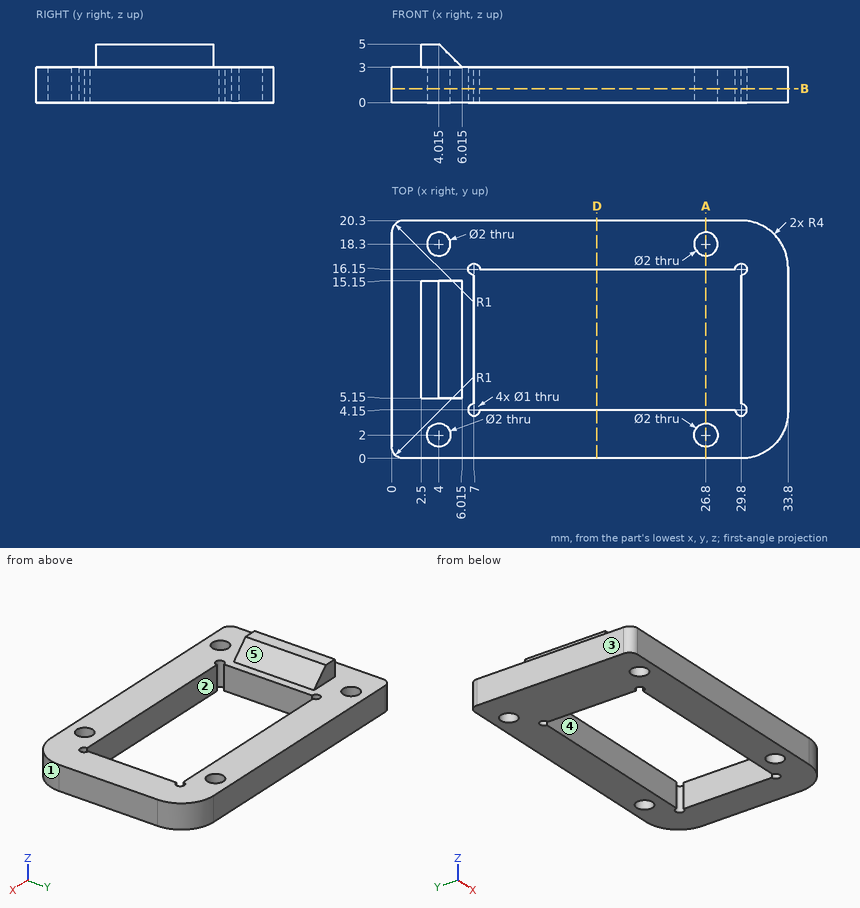
Here's the drawing with two shaded views (mm, measured from the low corner). I have some questions. A direction names the side the tool comes from. Coordinates: 2 decimals unless noted, no trailing zeros. Order: outer loops, then holes, each group sorted by start corner. A loop starts at its lowest first (then second) coordinate and runs counter-clockwise, first axis right, second up.
Item 1: Which directions (+Z, -Z, +X, -X, +Y, -Y) give clear straight access to the entire face, cutting with the end or side of a thin tool? Please do the marked faces 4 and 5.
Response values:
face 4: +Z, -Z
face 5: +Z, +X, +Y, -Y
Item 2: If we section it at A-A, the plane x = 26.8: List the corners of the cut face in (y, z) for me.
Response values:
outline: (0, 0) - (1, 0) - (1, 3) - (0, 3) - close; (3, 0) - (4.15, 0) - (4.15, 3) - (3, 3) - close; (16.15, 0) - (17.3, 0) - (17.3, 3) - (16.15, 3) - close; (19.3, 0) - (20.3, 0) - (20.3, 3) - (19.3, 3) - close
Item 3: I'm going to push flat-ended pins straight in: pin 1 Ø0.6 at (x, z) = (5, 4.5) entering from -Y; pin 2 Ø1 at (x, y) = (23.5, 16.5) entering from +Z; pin 3 Ø0.6 at (x, z) = (5, 4) entering from +Y; pin 4 Ø2 at (y, z) = (10.5, 4.5) entering from -X. Where does each tip first touch, or does it pass through?
Response values:
pin 1: passes through
pin 2: stops at z = 3
pin 3: stops at y = 15.15
pin 4: stops at x = 2.5
Item 4: Thinking about a two-plate mould opening in Y: for the marked faces 1, 2 and 3, which applies, pulls with the +Y half, pulls with the -Y half, needs draft (parallel to the pull), parting line crosses it, or undercut?
Response values:
face 1: pulls with the -Y half
face 2: undercut
face 3: needs draft
Item 5: I need wall thicknesses on probe 1 along Y at (x, z) = (26.8, 1.5); probe 2 along Y at (x, z) = (9, 2.7); probe 3 along X at (y, z) = (11.75, 1.15). Which ranges of each line are inside material? Lowest first, please.
Response values:
probe 1: y = 0 to 1, 3 to 4.15, 16.15 to 17.3, 19.3 to 20.3
probe 2: y = 0 to 4.15, 16.15 to 20.3
probe 3: x = 0 to 7, 29.8 to 33.8
Item 6: If we section it at B-B, the plane z = 1.2: List the corners of the cut face in (x, y) for me.
Response values:
outline: (0, 1) arc R1 ccw to (1, 0) - (29.8, 0) arc R4 ccw to (33.8, 4) - (33.8, 16.3) arc R4 ccw to (29.8, 20.3) - (1, 20.3) arc R1 ccw to (0, 19.3) - close; hole circle Ø2 at (4, 2); hole circle Ø2 at (4, 18.3); hole (7, 4.65) arc R0.5 ccw (long way) to (7.5, 4.15) - (29.3, 4.15) arc R0.5 ccw (long way) to (29.8, 4.65) - (29.8, 15.65) arc R0.5 ccw (long way) to (29.3, 16.15) - (7.5, 16.15) arc R0.5 ccw (long way) to (7, 15.65) - close; hole circle Ø2 at (26.8, 2); hole circle Ø2 at (26.8, 18.3)
Item 7: If we section it at D-D, the plane x = 17.5: List the corners of the cut face in (y, z) for me, then the cut area to 3 significant figures.
Response values:
outline: (0, 0) - (4.15, 0) - (4.15, 3) - (0, 3) - close; (16.15, 0) - (20.3, 0) - (20.3, 3) - (16.15, 3) - close
area: 24.9 mm2
